from build123d import *

# Parameters (mm, degrees)
CYLINDER086_R          = 12
CYLINDER086_DEPTH      = 26
BOX065_W               = 12
BOX065_H               = 12
BOX065_DEPTH           = 26
CYLINDER087_R          = 12
CYLINDER087_DEPTH      = 26
BOX066_W               = 12
BOX066_H               = 12
BOX066_DEPTH           = 26
CUT039_PLACEMENT_ANGLE = 90
CYLINDER088_R          = 12
CYLINDER088_DEPTH      = 26
BOX067_W               = 12
BOX067_H               = 12
BOX067_DEPTH           = 26
CUT040_PLACEMENT_ANGLE = 180
CYLINDER089_R          = 12
CYLINDER089_DEPTH      = 26
BOX068_W               = 12
BOX068_H               = 12
BOX068_DEPTH           = 26
CUT041_PLACEMENT_ANGLE = 90
BOX064_W               = 132
BOX064_H               = 105
BOX064_DEPTH           = 26
CYLINDER082_R          = 12
CYLINDER082_DEPTH      = 26
BOX060_W               = 12
BOX060_H               = 12
BOX060_DEPTH           = 26
CYLINDER083_R          = 12
CYLINDER083_DEPTH      = 26
BOX061_W               = 12
BOX061_H               = 12
BOX061_DEPTH           = 26
CUT034_PLACEMENT_ANGLE = 90
CYLINDER084_R          = 12
CYLINDER084_DEPTH      = 26
BOX062_W               = 12
BOX062_H               = 12
BOX062_DEPTH           = 26
CUT035_PLACEMENT_ANGLE = 180
CYLINDER085_R          = 12
CYLINDER085_DEPTH      = 26
BOX063_W               = 12
BOX063_H               = 12
BOX063_DEPTH           = 26
CUT036_PLACEMENT_ANGLE = 90
BOX059_W               = 140
BOX059_H               = 113
BOX059_DEPTH           = 26


with BuildPart() as cylinder088:
    # Cylinder086 → Cylinder086 (new body)
    with BuildSketch(Plane(origin=(12, 12, 0), x_dir=(1, 0, 0), z_dir=(0, 0, 1))):
        Circle(CYLINDER086_R)
    extrude(amount=CYLINDER086_DEPTH)


with BuildPart() as cutout014:
    # Box065 → Box065 (new body)
    with BuildSketch(Plane.XY):
        with Locations((6, 6)):
            Rectangle(BOX065_W, BOX065_H)
    extrude(amount=BOX065_DEPTH)

    # Cut038: cut Cylinder088
    add(cylinder088.part, mode=Mode.SUBTRACT)


with BuildPart() as cutout014_1:
    # Cut038 placement: moved
    add(cutout014.part.moved(Location((4, 4, 0))))


with BuildPart() as cylinder089:
    # Cylinder087 → Cylinder087 (new body)
    with BuildSketch(Plane(origin=(12, 12, 0), x_dir=(1, 0, 0), z_dir=(0, 0, 1))):
        Circle(CYLINDER087_R)
    extrude(amount=CYLINDER087_DEPTH)


with BuildPart() as cutout015:
    # Box066 → Box066 (new body)
    with BuildSketch(Plane.XY):
        with Locations((6, 6)):
            Rectangle(BOX066_W, BOX066_H)
    extrude(amount=BOX066_DEPTH)

    # Cut039: cut Cylinder089
    add(cylinder089.part, mode=Mode.SUBTRACT)


with BuildPart() as cutout015_1:
    # Cut039 placement: moved
    add(cutout015.part.moved(Location((136, 4, 0))).rotate(Axis((136, 4, 0), (0, 0, 1)), CUT039_PLACEMENT_ANGLE))


with BuildPart() as cylinder090:
    # Cylinder088 → Cylinder088 (new body)
    with BuildSketch(Plane(origin=(12, 12, 0), x_dir=(1, 0, 0), z_dir=(0, 0, 1))):
        Circle(CYLINDER088_R)
    extrude(amount=CYLINDER088_DEPTH)


with BuildPart() as cutout016:
    # Box067 → Box067 (new body)
    with BuildSketch(Plane.XY):
        with Locations((6, 6)):
            Rectangle(BOX067_W, BOX067_H)
    extrude(amount=BOX067_DEPTH)

    # Cut040: cut Cylinder090
    add(cylinder090.part, mode=Mode.SUBTRACT)


with BuildPart() as cutout016_1:
    # Cut040 placement: moved
    add(cutout016.part.moved(Location((136, 109, 0))).rotate(Axis((136, 109, 0), (0, 0, 1)), CUT040_PLACEMENT_ANGLE))


with BuildPart() as cylinder091:
    # Cylinder089 → Cylinder089 (new body)
    with BuildSketch(Plane(origin=(12, 12, 0), x_dir=(1, 0, 0), z_dir=(0, 0, 1))):
        Circle(CYLINDER089_R)
    extrude(amount=CYLINDER089_DEPTH)


with BuildPart() as cuts003:
    # Box068 → Box068 (new body)
    with BuildSketch(Plane.XY):
        with Locations((6, 6)):
            Rectangle(BOX068_W, BOX068_H)
    extrude(amount=BOX068_DEPTH)

    # Cut041: cut Cylinder091
    add(cylinder091.part, mode=Mode.SUBTRACT)


with BuildPart() as cuts003_1:
    # Cut041 placement: moved
    add(cuts003.part.moved(Location((4, 109, 0))).rotate(Axis((4, 109, 0), (0, 0, -1)), CUT041_PLACEMENT_ANGLE))

    # Fusion043: union cutOut014, cutOut015, cutOut016
    add(cutout014_1.part)
    add(cutout015_1.part)
    add(cutout016_1.part)


with BuildPart() as wallcut:
    # Box064 → Box064 (new body)
    with BuildSketch(Plane(origin=(4, 4, 0), x_dir=(1, 0, 0), z_dir=(0, 0, 1))):
        with Locations((66, 52.5)):
            Rectangle(BOX064_W, BOX064_H)
    extrude(amount=BOX064_DEPTH)

    # Cut042: cut cuts003
    add(cuts003_1.part, mode=Mode.SUBTRACT)


with BuildPart() as cylinder084:
    # Cylinder082 → Cylinder082 (new body)
    with BuildSketch(Plane(origin=(12, 12, 0), x_dir=(1, 0, 0), z_dir=(0, 0, 1))):
        Circle(CYLINDER082_R)
    extrude(amount=CYLINDER082_DEPTH)


with BuildPart() as cutout010:
    # Box060 → Box060 (new body)
    with BuildSketch(Plane.XY):
        with Locations((6, 6)):
            Rectangle(BOX060_W, BOX060_H)
    extrude(amount=BOX060_DEPTH)

    # Cut033: cut Cylinder084
    add(cylinder084.part, mode=Mode.SUBTRACT)


with BuildPart() as cylinder085:
    # Cylinder083 → Cylinder083 (new body)
    with BuildSketch(Plane(origin=(12, 12, 0), x_dir=(1, 0, 0), z_dir=(0, 0, 1))):
        Circle(CYLINDER083_R)
    extrude(amount=CYLINDER083_DEPTH)


with BuildPart() as cutout011:
    # Box061 → Box061 (new body)
    with BuildSketch(Plane.XY):
        with Locations((6, 6)):
            Rectangle(BOX061_W, BOX061_H)
    extrude(amount=BOX061_DEPTH)

    # Cut034: cut Cylinder085
    add(cylinder085.part, mode=Mode.SUBTRACT)


with BuildPart() as cutout011_1:
    # Cut034 placement: moved
    add(cutout011.part.moved(Location((140, 0, 0))).rotate(Axis((140, 0, 0), (0, 0, 1)), CUT034_PLACEMENT_ANGLE))


with BuildPart() as cylinder086:
    # Cylinder084 → Cylinder084 (new body)
    with BuildSketch(Plane(origin=(12, 12, 0), x_dir=(1, 0, 0), z_dir=(0, 0, 1))):
        Circle(CYLINDER084_R)
    extrude(amount=CYLINDER084_DEPTH)


with BuildPart() as cutout012:
    # Box062 → Box062 (new body)
    with BuildSketch(Plane.XY):
        with Locations((6, 6)):
            Rectangle(BOX062_W, BOX062_H)
    extrude(amount=BOX062_DEPTH)

    # Cut035: cut Cylinder086
    add(cylinder086.part, mode=Mode.SUBTRACT)


with BuildPart() as cutout012_1:
    # Cut035 placement: moved
    add(cutout012.part.moved(Location((140, 113, 0))).rotate(Axis((140, 113, 0), (0, 0, 1)), CUT035_PLACEMENT_ANGLE))


with BuildPart() as cylinder087:
    # Cylinder085 → Cylinder085 (new body)
    with BuildSketch(Plane(origin=(12, 12, 0), x_dir=(1, 0, 0), z_dir=(0, 0, 1))):
        Circle(CYLINDER085_R)
    extrude(amount=CYLINDER085_DEPTH)


with BuildPart() as cuts002:
    # Box063 → Box063 (new body)
    with BuildSketch(Plane.XY):
        with Locations((6, 6)):
            Rectangle(BOX063_W, BOX063_H)
    extrude(amount=BOX063_DEPTH)

    # Cut036: cut Cylinder087
    add(cylinder087.part, mode=Mode.SUBTRACT)


with BuildPart() as cuts002_1:
    # Cut036 placement: moved
    add(cuts002.part.moved(Location((0, 113, 0))).rotate(Axis((0, 113, 0), (0, 0, -1)), CUT036_PLACEMENT_ANGLE))

    # Fusion042: union cutOut010, cutOut011, cutOut012
    add(cutout010.part)
    add(cutout011_1.part)
    add(cutout012_1.part)


with BuildPart() as wall001:
    # Box059 → Box059 (new body)
    with BuildSketch(Plane.XY):
        with Locations((70, 56.5)):
            Rectangle(BOX059_W, BOX059_H)
    extrude(amount=BOX059_DEPTH)

    # Cut037: cut cuts002
    add(cuts002_1.part, mode=Mode.SUBTRACT)

    # Cut043: cut wallCut
    add(wallcut.part, mode=Mode.SUBTRACT)


solid = wall001.part
Work out the finished part from the listing and answer in its coordinate system (mm). A direction names the side the tool comes from. Give positions to 0.01 mm unless a question says otherwise; leave off trailing zeros. Write each loop counter-clockwise with the first axis right and the second up, starting at its lowest first coordinate (ties: lowest second). Pieces come first, ordered by that corner, then holes. Notation, with made-up numbers: M 89.5,-39.75 L 103.5,-39.75 A31 ccw 103.5,-8.75 Z; hole C 80.25,47.5 d7. An arc over 180 degrees is marked long. Answer as CSV lines item,"result".
Q1. Find the intervals of material crossed by probe 1 along Y at (x, z) = (24.5, 7.5); probe 2 along X at (y, z) = (28.5, 16); probe 3 along Y at (x, z) = (129.5, 6.75), in increasing order. Write a range as [from, to].
A:
probe 1,"y = [0, 4], [109, 113]"
probe 2,"x = [0, 4], [136, 140]"
probe 3,"y = [0.09, 5.33], [107.67, 112.91]"
Q2. The mould has two halves that part along X. Classify faces 3 (the cylindrical face through (3.61, 109.58, 12.82)), 4 (the flat face through (136, 56, 13)), 5 (the flat face through (69, 0, 13)): +X half, -X half, draft (parallel to the pull), parting line (faces both ways), or undercut.
A:
face 3,"-X half"
face 4,"undercut"
face 5,"draft"
Q3. A cutting plane is placed at C-C on x = 84.5. Write down the section's boundary in (y, z), plus the area to 3 significant figures.
A:
outline,"M 0,0 L 4,0 L 4,26 L 0,26 Z; M 109,0 L 113,0 L 113,26 L 109,26 Z"
area,"208 mm²"
Q4. A cutting plane is placed at B-B on z = 21. Write down the section's boundary in (x, y).
A:
outline,"M 0,12 A12 ccw 12,0 L 128,0 A12 ccw 140,12 L 140,101 A12 ccw 128,113 L 12,113 A12 ccw 0,101 Z; hole M 4,16 A12 ccw 16,4 L 124,4 A12 ccw 136,16 L 136,97 A12 ccw 124,109 L 16,109 A12 ccw 4,97 Z"
Q5. A cutting plane is placed at A-A on y = 68. Write down the section's boundary in (x, z), plus the area to 3 significant figures.
A:
outline,"M 0,0 L 4,0 L 4,26 L 0,26 Z; M 136,0 L 140,0 L 140,26 L 136,26 Z"
area,"208 mm²"
Q6. A tool of negligible diameter and unlimited length cuts with its end or side. For faces 1 (the cylindrical face through (3.42, 3.61, 12.82)), 2 (the cylindrical face through (132.39, 7.42, 12.82)), from which of +Z, -Z, +X, -X, +Y, -Y can it reach the whole face along a straight path? Write none if from no direction.
A:
face 1,"+Z, -Z, -X, -Y"
face 2,"+Z, -Z"
